Could you check a few things on this model? Use its own coordinates, in mm. A direction names the side the tool comes from. Give positions to 0.01 mm unless a question says otherwise; leave off trailing zeros. Loops run counter-clockwise (first coordinate to the right, second up) from the corner with the lowest first, then second, coordinate; pieces in that order, holes last. Notation, with made-up numbers: M -5.5,33.5 L 51.5,33.5 A26 cw 51.5,69.5 Z; hole C -27,26.5 d5. An arc over 180 degrees is marked long. Write each question's results on one line, items separated by ' | '. Start each with the question number.
from build123d import *

# Parameters (mm, degrees)
CROQUIS1_R                   = 1.5
SALIENTE_EXTRUIR1_DEPTH      = 3.5
CORTAR_EXTRUIR1_DEPTH        = 2
SALIENTE_EXTRUIR2_DEPTH      = 2.5
SALIENTE_EXTRUIR2_DEPTH_BACK = 3.5
CROQUIS3_R                   = 1.625
CROQUIS4_W                   = 4
CROQUIS4_H                   = 8.575
SALIENTE_EXTRUIR3_DEPTH      = 2.5
CORTAR_EXTRUIR2_DEPTH        = 2.5


with BuildPart() as part:
    # Croquis1 → Saliente-Extruir1 (new body)
    with BuildSketch(Plane.XY):
        Polygon((88.732371, -80.148646), (88.732371, -81.493646), (90.077371, -80.148646), (96.232371, -80.148646), (96.232371, -66.648646), (88.732371, -66.648646), align=None)
        with Locations((92.232371, -75.223646)):
            Circle(CROQUIS1_R, mode=Mode.SUBTRACT)
    extrude(amount=SALIENTE_EXTRUIR1_DEPTH)

    # Croquis2 → Cortar-Extruir1 (cut)
    with BuildSketch(Plane.XY.offset(3.5)):
        Polygon((92.232371, -72.053646), (89.48707047, -73.638646), (89.48707047, -76.808646), (92.232371, -78.393646), (94.97767153, -76.808646), (94.97767153, -73.638646), align=None)
    extrude(amount=-CORTAR_EXTRUIR1_DEPTH, mode=Mode.SUBTRACT)

    # Croquis3 → Saliente-Extruir2 (add, two sides: drawn at the far end of the back side and taken through both)
    with BuildSketch(Plane.XY.offset(3.5).offset(-SALIENTE_EXTRUIR2_DEPTH_BACK)):
        Polygon((88.732371, -81.493646), (75.732371, -81.493646), (75.732371, -74.071146), (83.98707047, -66.648646), (83.98707047, -75.223646), (87.98707047, -75.223646), (87.98707047, -66.648646), (88.732371, -66.648646), align=None)
        with Locations((79.72767153, -75.223646)):
            Circle(CROQUIS3_R, mode=Mode.SUBTRACT)
    extrude(amount=SALIENTE_EXTRUIR2_DEPTH + SALIENTE_EXTRUIR2_DEPTH_BACK)

    # Croquis4 → Saliente-Extruir3 (add)
    with BuildSketch(Plane.XY.offset(6)):
        with Locations((85.98707047, -70.936146)):
            Rectangle(CROQUIS4_W, CROQUIS4_H)
    extrude(amount=-SALIENTE_EXTRUIR3_DEPTH)

    # Croquis5 → Cortar-Extruir2 (cut)
    with BuildSketch(Plane.XY.offset(6)):
        Polygon((79.72767153, -78.393646), (82.47297206, -76.808646), (82.47297206, -73.638646), (79.72767153, -72.053646), (76.982371, -73.638646), (76.982371, -76.808646), align=None)
    extrude(amount=-CORTAR_EXTRUIR2_DEPTH, mode=Mode.SUBTRACT)


solid = part.part
1) Please list where these lines run through material, in increasing order: line 1 (X direction, y = -74.5, z = 1.15); line 2 (Z direction, x = 86.5, y = -68); line 3 (Z direction, x = 95.25, y = -75.25). Write a range as from..to.
2) I'm going to push flat-ended pins straight in: P1, Ø1, axis at x = 85.5, z = 1.5, coming from the +Y side; P2, Ø1.2, axis at x = 86, y = -73, coming from the -Z side; P3, Ø0.8, axis at y = -74.5, z = 4.5, coming from the +X side. Where does each tip first touch, or does it pass through?
3) Thinking about a two-plate mould opening in X: for faces 1 (the face through (90.879, -72.835, 2.514)), 2 (the face through (75.732, -78, 3)), 3 (the face through (82, -81.494, 3)), which applies, pulls with the +X half, pulls with the -X half, needs draft (parallel to the pull), parting line crosses it, or undercut?
4) If we section it at D-D on y = -79.5: Write out the boundary of the cut face in (x, z).
5) If we section it at A-A on z = 5: Write out the boundary of the cut face in (x, y), plus the area to 3 significant figures.
6) If we section it at B-B on x = 78.5: Write out the boundary of the cut face in (y, z), plus the area to 3 significant figures.
7) If we section it at C-C on z = 0.55: Write out the boundary of the cut face in (x, y) (3 decimals), plus the area to 3 significant figures.
8) Which directions (+Z, -Z, +X, -X, +Y, -Y) give clear straight access to the entire face, cutting with the end or side of a thin tool? Please do faces 4 (the face through (92, -72, 3.5)), 5 (the face through (90.84, -77.59, 2.51)), 6 (the face through (86, -75.224, 2)), 7 (the face through (93, -80.149, 2)).
Calculated:
1) line 1: x = 75.73..78.27, 81.18..83.99, 87.99..90.92, 93.55..96.23 | line 2: z = 3.5..6 | line 3: z = 0..3.5
2) P1: stops at y = -75.22 | P2: stops at z = 3.5 | P3: stops at x = 88.73
3) face 1: undercut | face 2: pulls with the -X half | face 3: needs draft
4) outline: M 75.73,0 L 96.23,0 L 96.23,3.5 L 88.73,3.5 L 88.73,6 L 75.73,6 Z
5) outline: M 75.73,-81.49 L 88.73,-81.49 L 88.73,-66.65 L 83.99,-66.65 L 75.73,-74.07 Z; hole M 76.98,-76.81 L 79.73,-78.39 L 82.47,-76.81 L 82.47,-73.64 L 79.73,-72.05 L 76.98,-73.64 Z | area: 136 mm2
6) outline: M -81.49,0 L -76.29,0 L -76.29,3.5 L -77.68,3.5 L -77.68,6 L -81.49,6 Z; M -74.16,0 L -71.58,0 L -71.58,6 L -72.76,6 L -72.76,3.5 L -74.16,3.5 Z | area: 39.7 mm2
7) outline: M 75.732,-81.494 L 88.732,-81.494 L 90.077,-80.149 L 96.232,-80.149 L 96.232,-66.649 L 87.987,-66.649 L 87.987,-75.224 L 83.987,-75.224 L 83.987,-66.649 L 75.732,-74.071 Z; hole C 79.728,-75.224 d3.25; hole C 92.232,-75.224 d3 | area: 215 mm2
8) face 4: +Z, +X, +Y, -Y | face 5: +Z | face 6: -Z, +Y | face 7: +Z, -Z, +X, -Y
